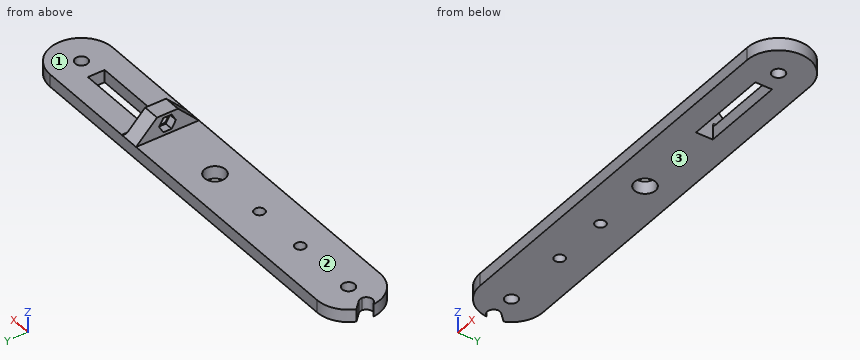
from build123d import *

# Parameters (mm, degrees)
ESQUISSE1_R             = 3
ESQUISSE1_R_2           = 5
ESQUISSE1_R_3           = 2.5
ESQUISSE1_W             = 40
ESQUISSE1_H             = 8
BOSS_EXTRU_1_DEPTH      = 6
ESQUISSE2_R             = 3
BOSS_EXTRU_2_DEPTH      = 8
CONG_2_R                = 2
ENL_V_MAT_EXTRU_1_DEPTH = 4
ENL_V_START             = -10
ENL_V_MAT_EXTRU_4_DEPTH = 10


with BuildPart() as part:
    # Esquisse1 → Boss.-Extru.1 (new body)
    with BuildSketch(Plane.XY):
        with BuildLine():
            Line((90, -15), (-90, -15))
            ThreePointArc((-90, -15), (-105, 0), (-90, 15))
            Line((-90, 15), (90, 15))
            ThreePointArc((90, 15), (105, 0), (90, -15))
        make_face()
        with Locations((90, 0)):
            Circle(ESQUISSE1_R, mode=Mode.SUBTRACT)
        with Locations(Location((-90, 0, 0), (0, 0, 180))):
            Circle(ESQUISSE1_R, mode=Mode.SUBTRACT)
        Circle(ESQUISSE1_R_2, mode=Mode.SUBTRACT)
        with Locations((-57.5, 0)):
            Circle(ESQUISSE1_R_3, mode=Mode.SUBTRACT)
        with Locations((-30, 0)):
            Circle(ESQUISSE1_R_3, mode=Mode.SUBTRACT)
        with Locations((60, 0)):
            Rectangle(ESQUISSE1_W, ESQUISSE1_H, mode=Mode.SUBTRACT)
    extrude(amount=BOSS_EXTRU_1_DEPTH)

    # Esquisse2 → Boss.-Extru.2 (add)
    with BuildSketch(Plane(origin=(40, 0, 0), x_dir=(0, 0, -1), z_dir=(1, 0, 0))):
        Polygon((-16, 5), (-16, -5), (-6, -15), (-6, -5), (-6, 5), (-6, 15), align=None)
        with Locations((-11, 0)):
            Circle(ESQUISSE2_R, mode=Mode.SUBTRACT)
    extrude(amount=-BOSS_EXTRU_2_DEPTH)

    # Congé2
    cong_2_edges = [part.edges().sort_by_distance(p)[0] for p in [
        (40, 9.5, 6),
        (40, -9.5, 6),
    ]]
    fillet(cong_2_edges, radius=CONG_2_R - 0.0001)  # a hair under: the kernel refuses the full size

    # Esquisse3 → Enlèv. mat.-Extru.1 (cut)
    with BuildSketch(Plane.ZY.offset(-32)):
        Polygon((11, 4), (14.464101615, 2), (14.464101615, -2), (11, -4), (7.535898385, -2), (7.535898385, 2), align=None)
    extrude(amount=-ENL_V_MAT_EXTRU_1_DEPTH, mode=Mode.SUBTRACT)

    # Esquisse4 → Enlèv. mat.-Extru.4 (cut)
    with BuildSketch(Plane.XY.offset(6).offset(ENL_V_START)):
        with BuildLine():
            ThreePointArc((-105, 0), (-104.771638598, -1.148050297), (-104.121320344, -2.121320344))
            Line((-104.121320344, -2.121320344), (-99.878679656, 2.121320344))
            ThreePointArc((-99.878679656, 2.121320344), (-103.148050297, 2.771638598), (-105, 0))
        make_face()
        with BuildLine():
            Line((-99.878679656, 2.121320344), (-104.121320344, -2.121320344))
            ThreePointArc((-104.121320344, -2.121320344), (-100.851949703, -2.771638598), (-99, 0))
            ThreePointArc((-99, 0), (-99.228361402, 1.148050297), (-99.878679656, 2.121320344))
        make_face()
        with BuildLine():
            ThreePointArc((-105, 0), (-103.148050297, 2.771638598), (-99.878679656, 2.121320344))
            Line((-99.878679656, 2.121320344), (-103.750652313, 5.993293))
            ThreePointArc((-103.750652313, 5.993293), (-104.68434174, 3.061063158), (-105, 0))
        make_face()
        with BuildLine():
            Line((-104.94364809, -1.298992597), (-104.121320344, -2.121320344))
            ThreePointArc((-104.121320344, -2.121320344), (-104.771638598, -1.148050297), (-105, 0))
            ThreePointArc((-105, 0), (-104.985905401, -0.650107165), (-104.94364809, -1.298992597))
        make_face()
        with BuildLine():
            ThreePointArc((-105, 0), (-104.771638598, -1.148050297), (-104.121320344, -2.121320344))
            Line((-104.121320344, -2.121320344), (-99.878679656, 2.121320344))
            ThreePointArc((-99.878679656, 2.121320344), (-103.148050297, 2.771638598), (-105, 0))
        make_face()
        with BuildLine():
            Line((-99.878679656, 2.121320344), (-104.121320344, -2.121320344))
            ThreePointArc((-104.121320344, -2.121320344), (-100.851949703, -2.771638598), (-99, 0))
            ThreePointArc((-99, 0), (-99.228361402, 1.148050297), (-99.878679656, 2.121320344))
        make_face()
    extrude(amount=ENL_V_MAT_EXTRU_4_DEPTH, mode=Mode.SUBTRACT)


solid = part.part
Model file for the job. Use its own axes, mm. Face numbers are marked on the shaded views. A direction names the side the tool comes from. Coordinates: 2 decimals unless noted, no trailing zeros. Write each loop counter-clockwise with the first axis right and the second up, starting at its lowest first coordinate (ties: lowest second). Pieces come first, ordered by that corner, then holes. Notation, with made-up numbers: (-2, 26.5) -> (14, 26.5) arc R28 cw to (14, 45.5) -> close; hole circle Ø9 at (72, 59.5). An arc over 180 degrees is marked (long way). One line per item, written item: value. Start each with the question number.
1) Slice it at D-D on y = 10. Write the cut outline in (x, z).
2) Slice it at A-A on x = 74. Write the cut outline in (y, z).
3) Flat gauge pins, fed straight in: pin 1 Ø5 at (y, z) = (-9, 11.5) entering from +X; pin 2 Ø8 at (x, y) = (90, 0) entering from -Z; pin 3 Ø8 at (x, y) = (-30, 0) entering from +Z; pin 4 Ø9.5 at (y, z) = (0, 11) entering from -X. Where does each tip first touch, or does it go through?
4) Slice it at C-C on x = 0. Write the cut outline in (y, z).
5) Probe probe 1 along Y at (x, z) = (41.5, 2); probe 2 along Y at (x, z) = (0, 2); probe 3 along Z at (x, y) = (-26.5, -3). List the from-to ranges inside material, lowest first.
6) Which spindle directions (+Z, -Z, +X, -X, +Y, -Y) get a long thin tool onto all of the face, cutting with end or side? Do the marked faces 1, 2 and 3. Say none if no direction does.
7) Slice it at B-B on z = 2. Write the cut outline in (x, y), then the cut area to 3 significant figures.
Answers follow:
1. outline: (-101.18, 0) -> (101.18, 0) -> (101.18, 6) -> (42, 6) arc R2 cw to (40, 8) -> (40, 11) -> (32, 11) -> (32, 6) -> (-101.18, 6) -> close
2. outline: (-15, 0) -> (-4, 0) -> (-4, 6) -> (-15, 6) -> close; (4, 0) -> (15, 0) -> (15, 6) -> (4, 6) -> close
3. pin 1: x = 40
3. pin 2: z = 0
3. pin 3: z = 6
3. pin 4: x = 32
4. outline: (-15, 0) -> (-5, 0) -> (-5, 6) -> (-15, 6) -> close; (5, 0) -> (15, 0) -> (15, 6) -> (5, 6) -> close
5. probe 1: -15 to -4, 4 to 15
5. probe 2: -15 to -5, 5 to 15
5. probe 3: 0 to 6
6. face 1: +Z, +X, +Y, -Y
6. face 2: +Z, -X, +Y, -Y
6. face 3: -Z, +X, -X, +Y, -Y
7. outline: (-104.94, -1.3) arc R15 ccw to (-90, -15) -> (90, -15) arc R15 ccw to (90, 15) -> (-90, 15) arc R15 ccw to (-103.75, 5.99) -> (-99.88, 2.12) arc R3 cw to (-104.12, -2.12) -> close; hole circle Ø6 at (-90, 0); hole circle Ø5 at (-57.5, 0); hole circle Ø5 at (-30, 0); hole circle Ø10 at (0, 0); hole (40, -4) -> (80, -4) -> (80, 4) -> (40, 4) -> close; hole circle Ø6 at (90, 0)
7. area: 5,580 mm2
